Read the model definition and answer for the solid it produces. Units are mm, in the model's axes. Face numbers are marked on the shaded views. A direction names the side the tool comes from. Give positions to 0.01 mm unless a question says otherwise; leave off trailing zeros. Order: outer loops, then holes, each group sorted by start corner. A loop starts at its lowest first (then second) coordinate and runs counter-clockwise, first axis right, second up. Notation, with made-up numbers: (76, 3) -> (134, 3) arc R20 cw to (134, 41) -> close; hole circle Ø4 at (24.5, 24). An arc over 180 degrees is marked (long way). Use one line per item in the form item = value.
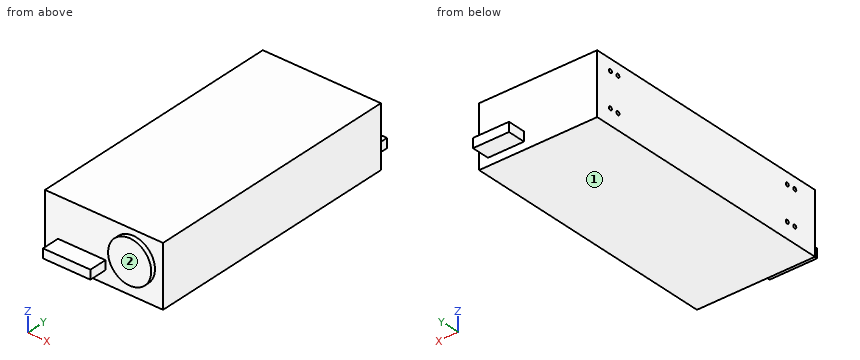
```python
from build123d import *

# Parameters (mm, degrees)
SKETCH_1_W          = 132
SKETCH_1_H          = 291
EXTRUDE_1_DEPTH     = 68
SKETCH_2_R          = 2
CUT_EXTRUDE_1_DEPTH = 4
SKETCH_3_W          = 53.053280534
SKETCH_3_H          = 10.202175613
EXTRUDE_2_DEPTH     = 20
SKETCH_4_R          = 24.120605075
EXTRUDE_3_DEPTH     = 5
SKETCH_5_W          = 40.253809201
SKETCH_5_H          = 10.422389964
EXTRUDE_4_DEPTH     = 20


with BuildPart() as part:
    # 草图1 → 凸台-拉伸1 (new body)
    with BuildSketch(Plane.XY):
        with Locations((-127.074626866, 141.649253731)):
            Rectangle(SKETCH_1_W, SKETCH_1_H)
    extrude(amount=EXTRUDE_1_DEPTH)

    # 草图2 → 切除-拉伸1 (cut)
    with BuildSketch(Plane.ZY.offset(193.074626866)):
        with Locations(Location((17.5, 23.149253731, 0), (0, 0, 270))):
            Circle(SKETCH_2_R)
        with Locations(Location((55.5, 23.149253731, 0), (0, 0, 270))):
            Circle(SKETCH_2_R)
        with Locations(Location((55.5, 33.149253731, 0), (0, 0, 270))):
            Circle(SKETCH_2_R)
        with Locations(Location((17.5, 33.149253731, 0), (0, 0, 270))):
            Circle(SKETCH_2_R)
        with Locations(Location((17.5, 269.449253731, 0), (0, 0, 90))):
            Circle(SKETCH_2_R)
        with Locations(Location((17.5, 259.449253731, 0), (0, 0, 90))):
            Circle(SKETCH_2_R)
        with Locations(Location((55.5, 259.449253731, 0), (0, 0, 90))):
            Circle(SKETCH_2_R)
        with Locations(Location((55.5, 269.449253731, 0), (0, 0, 90))):
            Circle(SKETCH_2_R)
    extrude(amount=-CUT_EXTRUDE_1_DEPTH, mode=Mode.SUBTRACT)

    # 草图3 → 凸台-拉伸2 (add)
    with BuildSketch(Plane.XZ.offset(3.850746269)):
        with Locations((-152.07170966, 19.120276631)):
            Rectangle(SKETCH_3_W, SKETCH_3_H)
    extrude(amount=EXTRUDE_2_DEPTH)

    # 草图4 → 凸台-拉伸3 (add)
    with BuildSketch(Plane.XZ.offset(3.850746269)):
        with Locations(Location((-94.251857707, 37.587190062, 0), (0, 0, 90))):
            Circle(SKETCH_4_R)
    extrude(amount=EXTRUDE_3_DEPTH)

    # 草图5 → 凸台-拉伸4 (add)
    with BuildSketch(Plane(origin=(0, 287.149253731, 0), x_dir=(1, 0, 0), z_dir=(0, 1, 0))):
        with Locations((-91.075289647, -13.720381028)):
            Rectangle(SKETCH_5_W, SKETCH_5_H)
    extrude(amount=EXTRUDE_4_DEPTH)


solid = part.part
```
Item 1: Which of the six approach directions +Z, -Z, +X, -X, +Y, -Y give full straight-line access (tool end or side, diameter ignored) to the marked faces 1 and 2?
Checks:
face_1 = -Z, +X, -X, +Y, -Y
face_2 = +Z, -Z, +X, -Y
Item 2: The part is cut by section B-B on z = 45. Give the vertices of the cut face in (x, y).
Checks:
outline = (-193.07, -3.85) -> (-117.21, -3.85) -> (-117.21, -8.85) -> (-71.3, -8.85) -> (-71.3, -3.85) -> (-61.07, -3.85) -> (-61.07, 287.15) -> (-193.07, 287.15) -> close
Item 3: Given pin 1 Ø2 at (x, z) = (-148.5, 23) entering from +Y; pin 2 Ø3.5 at (y, z) = (33.15, 55.5) entering from -X; pin 3 Ø3 at (y, z) = (295.5, 12.5) entering from -X, each flat-ended and moving along its own axis, determine where each tip first touches the part or whether it passes through.
Checks:
pin_1 = 287.15
pin_2 = -189.07
pin_3 = -111.2
Item 4: Straight lines are drawn through the part: L1, parallel to Y at x = -190, z = 17; L2, parallel to Y at x = -176, z = 11; L3, parallel to Z at x = -171, y = -4.5. For each, find the intervals that lie inside material, in ascending order. Write a range as from..to.
Checks:
L1 = -3.85..21.21, 25.09..31.21, 35.09..257.51, 261.39..267.51, 271.39..287.15
L2 = -3.85..287.15
L3 = 14.02..24.22
Item 5: The part is cut by section C-C on x = -89. Give the vertices of the cut face in (y, z), and give its area (3 significant figures).
Checks:
outline = (-8.85, 14.05) -> (-3.85, 14.05) -> (-3.85, 0) -> (287.15, 0) -> (287.15, 8.51) -> (307.15, 8.51) -> (307.15, 18.93) -> (287.15, 18.93) -> (287.15, 68) -> (-3.85, 68) -> (-3.85, 61.13) -> (-8.85, 61.13) -> close
area = 20,200 mm²
Item 6: The part is cut by section A-A on x = -143.5. Give the vertices of the cut face in (y, z), and give its area (3 significant figures).
Checks:
outline = (-23.85, 14.02) -> (-3.85, 14.02) -> (-3.85, 0) -> (287.15, 0) -> (287.15, 68) -> (-3.85, 68) -> (-3.85, 24.22) -> (-23.85, 24.22) -> close
area = 20,000 mm²
